Design review of the part built by this model. Coordinates are the model's own, in mm. A direction names the side the tool comes from. Give positions to 0.01 mm unless a question says otherwise; leave off trailing zeros. Write each loop counter-clockwise with the first axis right and the second up, starting at its lowest first coordinate (ties: lowest second). Pieces come first, ordered by that corner, then holes. Notation, with made-up numbers: (-32, 42.25) -> (24, 42.25) arc R20 ccw to (24, 68.25) -> close; hole circle Ø5 at (83.25, -16.5). An arc over 180 degrees is marked (long way). Put each result on its own line as item: value. Start each with the question number.
from build123d import *

# Parameters (mm, degrees)
F0_W     = 10
F0_H     = 15
F0_W_2   = 15
F0_H_2   = 10
F1_DEPTH = 45
F2_DEPTH = 35
F3_DEPTH = 17.5
F4_DEPTH = 7.5


with BuildPart() as f1:
    # F0 (on Right) → F1 (new body, symmetric)
    with BuildSketch(Plane.YZ):
        Polygon((0, 70), (0, 37.5), (10, 37.5), (10, 60), (10, 70), align=None)
        with Locations((5, 30)):
            Rectangle(F0_W, F0_H)
        Polygon((0, 22.5), (0, 0), (37.5, 0), (37.5, 10), (10, 10), (10, 22.5), align=None)
        Polygon((10, 37.5), (10, 22.5), (10, 10), (37.5, 10), (52.5, 10), (60, 10), (10, 60), align=None)
        with Locations((45, 5)):
            Rectangle(F0_W_2, F0_H_2)
        Polygon((52.5, 10), (52.5, 0), (70, 0), (70, 10), (60, 10), align=None)
    extrude(amount=F1_DEPTH, both=True)

    # F0 (on Right) → F2 (cut, symmetric)
    with BuildSketch(Plane.YZ):
        Polygon((10, 37.5), (10, 22.5), (10, 10), (37.5, 10), (52.5, 10), (60, 10), (10, 60), align=None)
    extrude(amount=F2_DEPTH, both=True, mode=Mode.SUBTRACT)

    # F0 (on Right) → F3 (cut, symmetric)
    with BuildSketch(Plane.YZ):
        with Locations((5, 30)):
            Rectangle(F0_W, F0_H)
    extrude(amount=F3_DEPTH, both=True, mode=Mode.SUBTRACT)

    # F0 (on Right) → F4 (cut, symmetric)
    with BuildSketch(Plane.YZ):
        with Locations((45, 5)):
            Rectangle(F0_W_2, F0_H_2)
    extrude(amount=F4_DEPTH, both=True, mode=Mode.SUBTRACT)


solid = f1.part
Q1. Take a section at B-B on z = 36. Give the boundary of the cut face in (x, y), then the cut area to 3 significant figures.
Q2. Take a section at A-A on x = 9. Give the boundary of the cut face in (y, z).
Q3. Mouldability with a two-part tool opening along Z and no side actions: class faces 1 (the face through (-35, 24, 24)), 2 (the face through (0, 5, 37.5)), 3 (the face through (-40, 35, 35)) as +Z half, -Z half, draft (parallel to the pull), parting line (faces both ways), or undercut.
Q4. Take a section at D-D on z = 20. Give the boundary of the cut face in (x, y).
Q5. Take a section at C-C on y = 12.5. Give the boundary of the cut face in (x, z), then the cut area to 3 significant figures.
Q6. To check wall thickness, follow probe 1 along Y at (x, z) = (7, 9); probe 2 along X at (y, z) = (39, 27); probe 3 along X at (y, z) = (44, 8). State the ranges of each line that lie inside material, in increasing order. Write a range as from..to.
Q7. Machinability: for faces 4 (the face through (1, 35, 0)), 5 (the face through (-7.5, 45, 5)), 6 (the face through (0, 5, 22.5)), 7 (the face through (35, 24, 24)), which of the approach directions +Z, -Z, +X, -X, +Y, -Y give a long, thin tool a straight path to every point of the face, cutting with its end or side? Answer none if there is none.
Q8. For pin 1 (5 mm diameter, centred on x = 3, z = 4, fed in from -Y); pin 2 (1.5 mm diameter, centred on x = 7.5, z = 50, fed in from +Y); pin 3 (18 mm diameter, centred on x = -5.5, y = 30, fed in from +Z), all flat-tipped, find the tip position at first contact; note any pin that passes through.
Result:
1. outline: (-45, 0) -> (-17.5, 0) -> (-17.5, 10) -> (-35, 10) -> (-35, 34) -> (-45, 34) -> close; (17.5, 0) -> (45, 0) -> (45, 34) -> (35, 34) -> (35, 10) -> (17.5, 10) -> close
1. area: 1,030 mm^2
2. outline: (0, 0) -> (70, 0) -> (70, 10) -> (10, 10) -> (10, 22.5) -> (0, 22.5) -> close; (0, 37.5) -> (10, 37.5) -> (10, 70) -> (0, 70) -> close
3. face 1: draft
3. face 2: undercut
3. face 3: +Z half
4. outline: (-45, 0) -> (45, 0) -> (45, 50) -> (35, 50) -> (35, 10) -> (-35, 10) -> (-35, 50) -> (-45, 50) -> close
5. outline: (-45, 0) -> (45, 0) -> (45, 57.5) -> (35, 57.5) -> (35, 10) -> (-35, 10) -> (-35, 57.5) -> (-45, 57.5) -> close
5. area: 1,850 mm^2
6. probe 1: y = 0..37.5, 52.5..70
6. probe 2: x = -45..-35, 35..45
6. probe 3: x = -45..-7.5, 7.5..45
7. face 4: -Z, +X, -X, +Y, -Y
7. face 5: +Z, -Z
7. face 6: +Y, -Y
7. face 7: +Z, +Y
8. pin 1: stops at y = 0
8. pin 2: stops at y = 10
8. pin 3: stops at z = 10
